from build123d import *

# Parameters (mm, degrees)
SKETCH2_R          = 12.7
SKETCH2_R_2        = 3.625
CUT_EXTRUDE1_DEPTH = 1
CUT_EXTRUDE2_DEPTH = 9.525


with BuildPart() as part:
    # Sketch1 → Revolve1 (revolve)
    with BuildSketch(Plane(origin=(0, 0, 0), x_dir=(0, 0, -1), z_dir=(1, 0, 0))):
        with BuildLine():
            Line((0, 25.4), (0, 2))
            Line((0, 2), (22.225, 2))
            Line((22.225, 2), (22.225, 25.4))
            ThreePointArc((22.225, 25.4), (11.1125, 34.925), (0, 25.4))
        make_face()
    revolve(axis=Axis((0, 0, -22.225), (0, 0, 1)))

    # Sketch2 → Cut-Extrude1 (cut)
    with BuildSketch(Plane.XY):
        Circle(SKETCH2_R)
        Circle(SKETCH2_R_2, mode=Mode.SUBTRACT)
    extrude(amount=-CUT_EXTRUDE1_DEPTH, mode=Mode.SUBTRACT)

    # Sketch3 → Cut-Extrude2 (cut)
    with BuildSketch(Plane.XY.offset(-1)):
        with BuildLine():
            Line((-0.459525068, 4.600054071), (-3.634525068, 11.337002474))
            ThreePointArc((-3.634525068, 11.337002474), (-3.603998477, 11.825642279), (-3.175, 12.061568196))
            Line((-3.175, 12.061568196), (3.175, 12.061568196))
            ThreePointArc((3.175, 12.061568196), (3.603998477, 11.825642279), (3.634525068, 11.337002474))
            Line((3.634525068, 11.337002474), (0.459525068, 4.600054071))
            ThreePointArc((0.459525068, 4.600054071), (0, 4.308619792), (-0.459525068, 4.600054071))
        make_face()
        with BuildLine():
            Line((3.577662719, 2.927796135), (10.58646865, 5.446474006))
            ThreePointArc((10.58646865, 5.446474006), (10.91040361, 5.813580085), (10.773880693, 6.283752633))
            Line((10.773880693, 6.283752633), (6.283752633, 10.773880693))
            ThreePointArc((6.283752633, 10.773880693), (5.813580085, 10.91040361), (5.446474006, 10.58646865))
            Line((5.446474006, 10.58646865), (2.927796135, 3.577662719))
            ThreePointArc((2.927796135, 3.577662719), (3.046654273, 3.046654273), (3.577662719, 2.927796135))
        make_face()
        with BuildLine():
            Line((4.600054071, -0.459525068), (11.337002474, -3.634525068))
            ThreePointArc((11.337002474, -3.634525068), (11.825642279, -3.603998477), (12.061568196, -3.175))
            Line((12.061568196, -3.175), (12.061568196, 3.175))
            ThreePointArc((12.061568196, 3.175), (11.825642279, 3.603998477), (11.337002474, 3.634525068))
            Line((11.337002474, 3.634525068), (4.600054071, 0.459525068))
            ThreePointArc((4.600054071, 0.459525068), (4.308619792, 0), (4.600054071, -0.459525068))
        make_face()
        with BuildLine():
            Line((2.927796135, -3.577662719), (5.446474006, -10.58646865))
            ThreePointArc((5.446474006, -10.58646865), (5.813580085, -10.91040361), (6.283752633, -10.773880693))
            Line((6.283752633, -10.773880693), (10.773880693, -6.283752633))
            ThreePointArc((10.773880693, -6.283752633), (10.91040361, -5.813580085), (10.58646865, -5.446474006))
            Line((10.58646865, -5.446474006), (3.577662719, -2.927796135))
            ThreePointArc((3.577662719, -2.927796135), (3.046654273, -3.046654273), (2.927796135, -3.577662719))
        make_face()
        with BuildLine():
            Line((-0.459525068, -4.600054071), (-3.634525068, -11.337002474))
            ThreePointArc((-3.634525068, -11.337002474), (-3.603998477, -11.825642279), (-3.175, -12.061568196))
            Line((-3.175, -12.061568196), (3.175, -12.061568196))
            ThreePointArc((3.175, -12.061568196), (3.603998477, -11.825642279), (3.634525068, -11.337002474))
            Line((3.634525068, -11.337002474), (0.459525068, -4.600054071))
            ThreePointArc((0.459525068, -4.600054071), (0, -4.308619792), (-0.459525068, -4.600054071))
        make_face()
        with BuildLine():
            Line((-3.577662719, -2.927796135), (-10.58646865, -5.446474006))
            ThreePointArc((-10.58646865, -5.446474006), (-10.91040361, -5.813580085), (-10.773880693, -6.283752633))
            Line((-10.773880693, -6.283752633), (-6.283752633, -10.773880693))
            ThreePointArc((-6.283752633, -10.773880693), (-5.813580085, -10.91040361), (-5.446474006, -10.58646865))
            Line((-5.446474006, -10.58646865), (-2.927796135, -3.577662719))
            ThreePointArc((-2.927796135, -3.577662719), (-3.046654273, -3.046654273), (-3.577662719, -2.927796135))
        make_face()
        with BuildLine():
            Line((-4.600054071, 0.459525068), (-11.337002474, 3.634525068))
            ThreePointArc((-11.337002474, 3.634525068), (-11.825642279, 3.603998477), (-12.061568196, 3.175))
            Line((-12.061568196, 3.175), (-12.061568196, -3.175))
            ThreePointArc((-12.061568196, -3.175), (-11.825642279, -3.603998477), (-11.337002474, -3.634525068))
            Line((-11.337002474, -3.634525068), (-4.600054071, -0.459525068))
            ThreePointArc((-4.600054071, -0.459525068), (-4.308619792, 0), (-4.600054071, 0.459525068))
        make_face()
        with BuildLine():
            Line((-2.927796135, 3.577662719), (-5.446474006, 10.58646865))
            ThreePointArc((-5.446474006, 10.58646865), (-5.813580085, 10.91040361), (-6.283752633, 10.773880693))
            Line((-6.283752633, 10.773880693), (-10.773880693, 6.283752633))
            ThreePointArc((-10.773880693, 6.283752633), (-10.91040361, 5.813580085), (-10.58646865, 5.446474006))
            Line((-10.58646865, 5.446474006), (-3.577662719, 2.927796135))
            ThreePointArc((-3.577662719, 2.927796135), (-3.046654273, 3.046654273), (-2.927796135, 3.577662719))
        make_face()
    extrude(amount=-CUT_EXTRUDE2_DEPTH, mode=Mode.SUBTRACT)


solid = part.part
Design review of the part built by this model. Coordinates are the model's own, in mm. A direction names the side the tool comes from. Coordinates: 2 decimals unless noted, no trailing zeros. Loops run counter-clockwise (first coordinate to the right, second up) from the corner with the lowest first, then second, coordinate; pieces in that order, holes last.
Item 1: Add section B-B (z = -6.75). Give the number of separate pieces and of enclosed holes in the cut face, and give its area (3 significant figures).
Completed:
separate pieces: 1
enclosed holes: 9
area: 3,360 mm2
Item 2: Draft analysis for pull direction X (two halves, no side actions). For faces 1 (the flat face through (0, -5, -22.225)), 2 (the flat face through (4.205, 7.131, -5.696)), state which applies: pulls with the +X half, pulls with the -X half, needs draft (parallel to the pull), parting line crosses it, or undercut.
Completed:
face 1: needs draft
face 2: undercut
Item 3: Add section A-A (z = -20.25). Write out the cut boundary in (x, y).
Completed:
outline: circle Ø60.47 at (0, 0); hole circle Ø4 at (0, 0)
Item 4: For faces 3 (the flat face through (-2.025, 7.921, -5.696)), 4 (the flat face through (-12, 5, 0)), list the 3-axis set-ups (+Z, -Z, +X, -X, +Y, -Y) from which the entire face can be reached by the end or side of a thin tool; tool diameter is ignored.
Completed:
face 3: +Z
face 4: +Z, +X, -X, +Y, -Y
Item 5: Clearance check with flat-ended pins moving along their axes: pin 1 (1.5 mm diameter, centred on x = -23, z = -20, fed in from -Y); pin 2 (3.5 mm diameter, centred on x = 9.5, y = 0, fed in from +Z) (3 decimals); pin 3 (5 mm diameter, centred on y = 8.5, z = -11.5, fed in from +X); pin 4 (2.5 mm diameter, centred on x = 0, y = 0, fed in from -Z). State where each tip first meets the part, or that it passes through.
Completed:
pin 1: stops at y = -21.68
pin 2: stops at z = -10.525
pin 3: stops at x = 34.4
pin 4: passes through
Item 6: Add section C-C (z = -14.75). Write out the cut boundary in (x, y), and give its area (3 significant figures).
Completed:
outline: circle Ø68.64 at (0, 0); hole circle Ø4 at (0, 0)
area: 3,690 mm2
Item 7: Wall thickness on L1, parallel to Z at x = -10.5, y = -4.5 (3 decimals); L2, parallel to Y at x = -9, z = -4; L3, parallel to Y at x = 0, z = -0.75 (3 decimals): over which ranges is each line inside the solid? List them lowest first.
Completed:
L1: z = -22.225 to -1
L2: y = -31.11 to -8.06, -4.88 to -2.53, 2.53 to 4.88, 8.06 to 31.11
L3: y = -28.046 to -12.7, -3.625 to -2, 2 to 3.625, 12.7 to 28.046
